Check sheet for the drawn part. Datum: minimum x, y, z corner. Units: mm. Give positions to 0.01 mm unless a question says otherwise; leave off trailing zeros. Loops run counter-clockwise (first coordinate to the right, second up) from the corner with the lowest first, then second, coordinate; pieces in that order, holes last. Notation, with made-up numbers: (42, 87.25) -> (79, 87.25) arc R23 ccw to (79, 96.25) -> close; hole circle Ø1 at (-21.75, 85). An arc over 180 degrees is marked (long way). One line per question, with ' | ' between items.
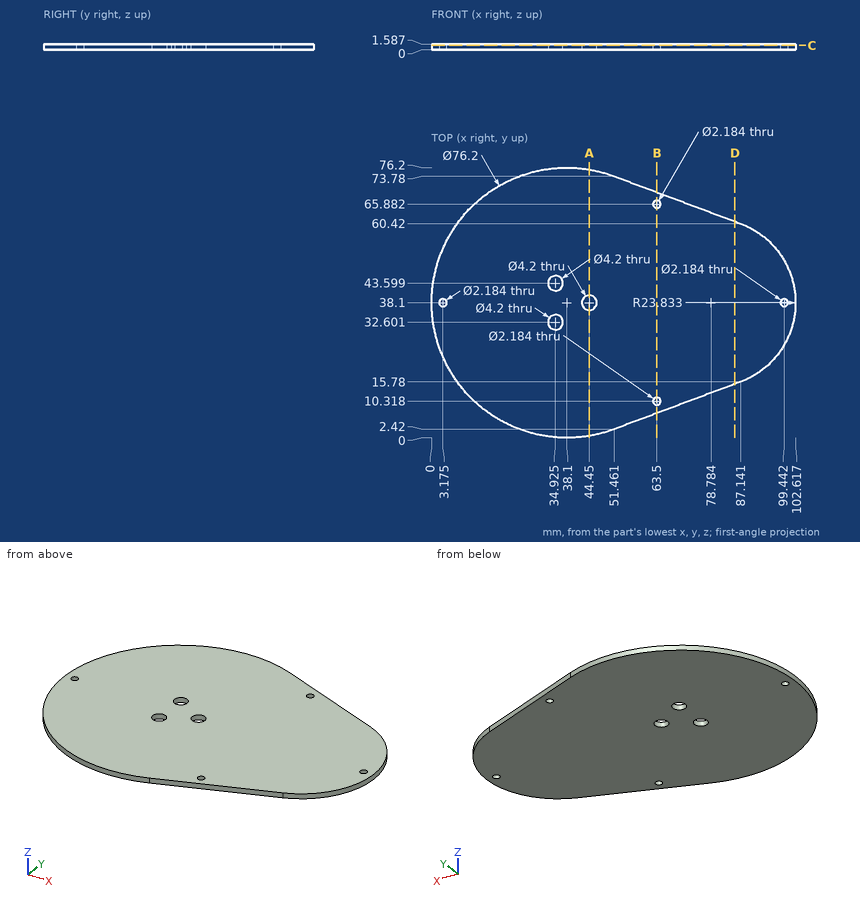
Item 1: Sectioned sample at A-A (x = 44.45). Record the cut outline in (y, z).
Result:
outline: (0.53, 0) -> (36, 0) -> (36, 1.59) -> (0.53, 1.59) -> close; (40.2, 0) -> (75.67, 0) -> (75.67, 1.59) -> (40.2, 1.59) -> close
Item 2: Scan lines: probe 1 along Y at (x, z) = (63.5, 1.15) (1 decimal); probe 2 along Y at (x, z) = (44.45, 0.9); probe 3 along X at (y, z) = (31.5, 0.45) (1 decimal). Record each from-to range of solid material in increasing order.
Result:
probe 1: 6.9 to 9.2, 11.4 to 64.8, 67 to 69.3 | probe 2: 0.53 to 36, 40.2 to 75.67 | probe 3: 0.6 to 33.1, 36.7 to 101.7
Item 3: Sectioned sample at D-D (x = 85.5). Record the cut outline in (y, z) (1 decimal).
Result:
outline: (15.2, 0) -> (61, 0) -> (61, 1.6) -> (15.2, 1.6) -> close
Item 4: Sectioned sample at B-B (x = 63.5). Record the cut outline in (y, z) (1 decimal).
Result:
outline: (6.9, 0) -> (9.2, 0) -> (9.2, 1.6) -> (6.9, 1.6) -> close; (11.4, 0) -> (64.8, 0) -> (64.8, 1.6) -> (11.4, 1.6) -> close; (67, 0) -> (69.3, 0) -> (69.3, 1.6) -> (67, 1.6) -> close
Item 5: Sectioned sample at C-C (z = 1.2). Give the number of separate pieces and of enclosed holes in the cut face, plus the area to 3 significant figures.
Result:
separate pieces: 1 | enclosed holes: 7 | area: 5,790 mm2
